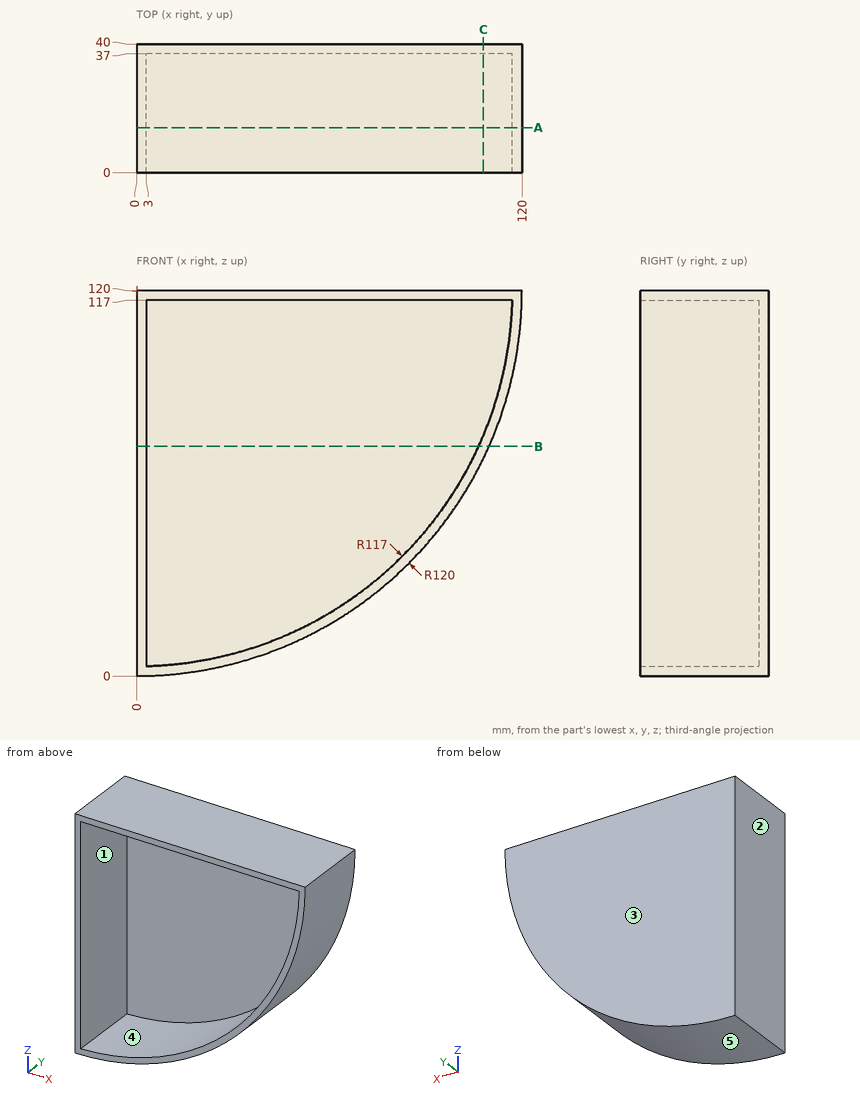
Part print with two shaded views. Sizes in mm from the minimum x, y, z corner. A direction names the side the tool comes from. Round coordinates to 2 decimals unless told otherwise and drop trailing zeros. Order: outer loops, then holes, each group sorted by start corner. A loop starts at its lowest first (then second) coordinate and runs counter-clockwise, first axis right, second up. Notation, with made-up numbers: (66.25, 29.25) - (97.25, 29.25) arc R19 ccw to (97.25, 33.25) - close; hole circle Ø6 at (-21, -11.5). An arc over 180 degrees is marked (long way). Answer in a Markdown table with one row per item. Add a question column.
(1) Band-saw the part on B-B on z = 71.5. List the corners of the cut face in (x, y).
(2) Probe L1, parallel to Y at x = 47, z = 109; L2, parallel to Z at x = 22, y = 23.5; L3, parallel to X at y = 2.5, z = 47. List the from-to ranges inside material, lowest first. Write a range as [from, to].
(3) Band-saw the part on A-A on y = 14. List the corners of the cut face in (x, z), and give its area (3 significant figures).
(4) Mould opens along X. For the marked faces 3, 4 and 5 say: +X half, -X half, draft (parallel to the pull), parting line (faces both ways), or undercut.
(5) Drop flat-ended pins along their axis: pin 1 Ø8 at (y, z) = (26, 14.5) entering from +X; pin 2 Ø4 at (y, z) = (33.5, 61) entering from -X; pin 3 Ø18.5 at (y, z) = (21.5, 48.5) entering from +X; pin 4 Ø8 at (x, z) = (85, 100.5) entering from -Y. Give the stop position or say it passes through.
(6) 3-axis set-ups, long thin cutter, end or side, ignore diameter. For the marked faces 1 and 2: which of +Z, -Z, +X, -X, +Y, -Y reach the whole face in a straight line?
(7) Band-saw the part on C-C on x = 108. List the corners of the cut face in (y, z).
Data:
| question | item | result |
|---|---|---|
| 1 | outline | (0, 0) - (3, 0) - (3, 37) - (106.47, 37) - (106.47, 0) - (109.76, 0) - (109.76, 40) - (0, 40) - close |
| 2 | L1 | y = [37, 40] |
| 2 | L2 | z = [2.03, 5.09], [117, 120] |
| 2 | L3 | x = [0, 3], [91.43, 95.24] |
| 3 | outline | (0, 0) arc R120 ccw to (120, 120) - (0, 120) - close; hole (3, 3.04) arc R117 ccw to (116.96, 117) - (3, 117) - close |
| 3 | area | 1,250 mm^2 |
| 4 | face 3 | draft |
| 4 | face 4 | undercut |
| 4 | face 5 | +X half |
| 5 | pin 1 | stops at x = 64.01 |
| 5 | pin 2 | stops at x = 0 |
| 5 | pin 3 | stops at x = 102.59 |
| 5 | pin 4 | stops at y = 37 |
| 6 | face 1 | -Y |
| 6 | face 2 | +Z, -Z, -X, +Y, -Y |
| 7 | outline | (0, 67.69) - (40, 67.69) - (40, 120) - (0, 120) - (0, 117) - (37, 117) - (37, 75) - (0, 75) - close |
